Could you check a few things on this model? Use its own coordinates, in mm. Round coordinates to 2 decimals unless told otherwise and drop trailing zeros. Loops run counter-clockwise (first coordinate to the right, second up) from the corner with the lowest first, then second, coordinate; pieces in that order, holes last. Notation, with made-up numbers: M -7.75,46 L 12.25,46 A18 ccw 12.25,59 Z; hole C 89,34 d6. An arc over 180 degrees is marked long. Return JSON: item names as keys, results as strings. Group by question number.
```python
from build123d import *

# Parameters (mm, degrees)
SKETCH_2_W           = 26
SKETCH_2_H           = 52
EXTRUDE_1_DEPTH      = 3
SKETCH_4_R           = 8
CUT_EXTRUDE_2_DEPTH  = 30.223278392
FILLET_1_R           = 2.6
SKETCH_3_R           = 2.75
CUT_EXTRUDE_16_DEPTH = 30.223278392


with BuildPart() as part:
    # 草图2 → 凸台-拉伸1 (new body)
    with BuildSketch(Plane.XY):
        Rectangle(SKETCH_2_W, SKETCH_2_H)
    extrude(amount=EXTRUDE_1_DEPTH)

    # 草图4 → 切除-拉伸2 (cut, through all)
    with BuildSketch(Plane.XY.offset(3)):
        Circle(SKETCH_4_R)
    extrude(amount=-CUT_EXTRUDE_2_DEPTH, mode=Mode.SUBTRACT)

    # 圆角1
    fillet_1_edges = [part.edges().sort_by_distance(p)[0] for p in [
        (-13, -26, 1.5),
        (-13, 26, 1.5),
        (13, 26, 1.5),
        (13, -26, 1.5),
    ]]
    fillet(fillet_1_edges, radius=FILLET_1_R)

    # 草图3 → 16 (cut, through all)
    with BuildSketch(Plane.XY.offset(3)):
        with Locations((0, 20)):
            Circle(SKETCH_3_R)
        with Locations(Location((0, -20, 0), (0, 0, 180))):
            Circle(SKETCH_3_R)
    extrude(amount=-CUT_EXTRUDE_16_DEPTH, mode=Mode.SUBTRACT)


solid = part.part
```
1. If we section it at C-C, the plane x = -4.25: Please give me the cut outline in (y, z), then the cut area to 3 significant figures.
2. If we section it at D-D, the plane z = 1.1: Please give me the cut outline in (x, y).
3. If we section it at A-A, the plane x = 0: Please give me the cut outline in (y, z), then the cut area to 3 significant figures.
4. If we section it at B-B, the plane y = 20: Please give me the cut outline in (x, z), then the cut area to 3 significant figures.
5. We'd pull the mould along X, two halves only. Please class faces 1 (the face through (-1.73, -7.81, 1.52)), 2 (the face through (0, 26, 1)), 3 (the face through (-12.259, -25.218, 1.521)): +X half, -X half, draft (parallel to the pull), parting line (faces both ways), or undercut.
6. I'm going to push flat-ended pins straight in: pin 1 Ø7 at (x, y) = (0, 20) entering from +Z; pin 2 Ø3.5 at (x, y) = (0, -20) entering from +Z. Where does each tip first touch, or does it pass through?
7. I need wall thicknesses on probe 1 along X at (y, z) = (-20, 2.2); probe 2 along Y at (x, z) = (0, 1.6); probe 3 along Y at (x, z) = (5, 2.2) (3 decimals). Which ranges of each line are inside material? Lowest first, please.
Geometry results:
{
 "1": {"outline": "M -26,0 L -6.78,0 L -6.78,3 L -26,3 Z; M 6.78,0 L 26,0 L 26,3 L 6.78,3 Z", "area": "115 mm^2"},
 "2": {"outline": "M -13,-23.4 A2.6 ccw -10.4,-26 L 10.4,-26 A2.6 ccw 13,-23.4 L 13,23.4 A2.6 ccw 10.4,26 L -10.4,26 A2.6 ccw -13,23.4 Z; hole C 0,0 d16; hole C 0,-20 d5.5; hole C 0,20 d5.5"},
 "3": {"outline": "M -26,0 L -22.75,0 L -22.75,3 L -26,3 Z; M -17.25,0 L -8,0 L -8,3 L -17.25,3 Z; M 8,0 L 17.25,0 L 17.25,3 L 8,3 Z; M 22.75,0 L 26,0 L 26,3 L 22.75,3 Z", "area": "75.0 mm^2"},
 "4": {"outline": "M -13,0 L -2.75,0 L -2.75,3 L -13,3 Z; M 2.75,0 L 13,0 L 13,3 L 2.75,3 Z", "area": "61.5 mm^2"},
 "5": {"face 1": "undercut", "face 2": "draft", "face 3": "-X half"},
 "6": {"pin 1": "z = 3", "pin 2": "through"},
 "7": {"probe 1": "-13 to -2.75, 2.75 to 13", "probe 2": "-26 to -22.75, -17.25 to -8, 8 to 17.25, 22.75 to 26", "probe 3": "-26 to -6.245, 6.245 to 26"}
}
